from build123d import *

# Parameters (mm, degrees)
CHAMFER1_SIZE      = 0.508
CHAMFER2_SIZE      = 1.524
CUT_EXTRUDE1_DEPTH = 30.6672
FILLET1_R          = 0.762


with BuildPart() as part:
    # Sketch1 → Revolve1 (revolve)
    with BuildSketch(Plane.XY):
        with BuildLine():
            Line((0, 26.543), (0, -20.066))
            Line((0, -20.066), (-6.35, -20.066))
            Line((-6.35, -20.066), (-6.35, -3.81))
            Line((-6.35, -3.81), (-5.1943, -3.81))
            Line((-5.1943, -3.81), (-5.1943, -1.27))
            ThreePointArc((-5.1943, -1.27), (-5.566274388, -0.371974388), (-6.4643, 0))
            Line((-6.4643, 0), (-11.43, 0))
            Line((-11.43, 0), (-11.43, 9.6012))
            Line((-11.43, 9.6012), (-7.874, 9.6012))
            Line((-7.874, 9.6012), (-7.874, 17.0942))
            ThreePointArc((-7.874, 17.0942), (-6.35, 19.4056), (-7.874, 21.717))
            Line((-7.874, 21.717), (-7.874, 23.749))
            Line((-7.874, 23.749), (-5.08, 26.543))
            Line((-5.08, 26.543), (0, 26.543))
        make_face()
    revolve(axis=Axis((0, -20.066, 0), (0, -1, 0)))

    # Chamfer1
    chamfer1_edges = [part.edges().sort_by_distance(p)[0] for p in [
        (11.43, 9.6012, 0),
        (11.43, 0, 0),
    ]]
    chamfer(chamfer1_edges, length=CHAMFER1_SIZE)

    # Chamfer2
    chamfer2_edges = [part.edges().sort_by_distance(p)[0] for p in [
        (6.35, -20.066, 0),
    ]]
    chamfer(chamfer2_edges, length=CHAMFER2_SIZE)

    # Sketch2 → Cut-Extrude1 (cut, through all)
    with BuildSketch(Plane(origin=(0, 9.6012, 0), x_dir=(1, 0, 0), z_dir=(0, 1, 0))):
        with BuildLine():
            Line((-9.398, 6.505574225), (-9.398, -6.505574225))
            ThreePointArc((-9.398, -6.505574225), (-11.43, 0), (-9.398, 6.505574225))
        make_face()
        with BuildLine():
            Line((9.398, 6.505574225), (9.398, -6.505574225))
            ThreePointArc((9.398, -6.505574225), (11.43, 0), (9.398, 6.505574225))
        make_face()
    extrude(amount=-CUT_EXTRUDE1_DEPTH, mode=Mode.SUBTRACT)

    # Fillet1
    fillet1_edges = [part.edges().sort_by_distance(p)[0] for p in [
        (7.874, 9.6012, 0),
    ]]
    fillet(fillet1_edges, radius=FILLET1_R)


solid = part.part
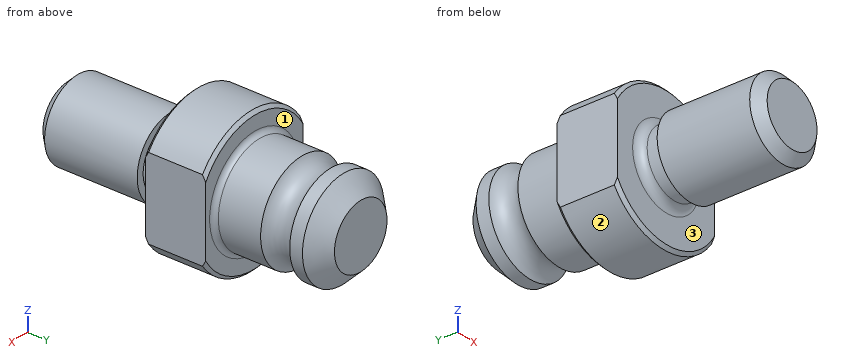
Design review of the part built by this model. Coordinates are the model's own, in mm. Face numbers are marked on the shaded views. A direction names the side the tool comes from. Coordinates: 2 decimals unless noted, no trailing zeros. Order: outer loops, then holes, each group sorted by start corner. A loop starts at its lowest first (then second) coordinate and runs counter-clockwise, first axis right, second up. Notation, with made-up numbers: M -33.75,40 L 15.25,40 A29 ccw 15.25,62 Z; hole C 85,30 d8. An arc over 180 degrees is marked long. Use a Markdown table: item, result.
(1) Add section C-C (y = -15.5). Give the boundary of the cut face in (x, z), then the cut area to 3 significant figures.
Worked answers:
| item | result |
|---|---|
| outline | C 0,0 d12.7 |
| area | 127 mm2 |
(2) Wall thickness on probe 1 along Y at (x, z) = (8, -5.5); probe 2 along Y at (x, z) = (-6.25, 0.75); probe 3 along Y at (x, z) = (3.5, 4): over which ranges is each line inside the solid? List them lowest first.
Worked answers:
| item | result |
|---|---|
| probe 1 | y = 0 to 9.6 |
| probe 2 | y = -18.6 to -3.81, -0.01 to 25.33 |
| probe 3 | y = -19.58 to -3.81, -0.73 to 26.31 |
(3) For P1, Ø8, axis at x = -4, y = -1.5, coming from the +Z side; P2, Ø1.5, axis at x = -7, z = -8, coming from the +Y side; P3, Ø1, axis at x = -4.5, z = -7, coming from the -Y side, all flat-tipped, find the tip position at first contact; note any pin that passes through.
Worked answers:
| item | result |
|---|---|
| P1 | stops at z = 11.42 |
| P2 | stops at y = 9.6 |
| P3 | stops at y = 0 |
(4) For the marked faces 1, 2 and 3, list the 3-axis set-ups (+Z, -Z, +X, -X, +Y, -Y) from which the entire face can be reached by the end or side of a thin tool; tool diameter is ignored.
Worked answers:
| item | result |
|---|---|
| face 1 | +Y |
| face 2 | -Z, +Y, -Y |
| face 3 | -Y |
(5) Add section B-B (z = 0). Give the boundary of the cut face in (x, y).
Worked answers:
| item | result |
|---|---|
| outline | M -9.4,0 L -6.46,0 A1.27 cw -5.19,-1.27 L -5.19,-3.81 L -6.35,-3.81 L -6.35,-18.54 L -4.83,-20.07 L 4.83,-20.07 L 6.35,-18.54 L 6.35,-3.81 L 5.19,-3.81 L 5.19,-1.27 A1.27 cw 6.46,0 L 9.4,0 L 9.4,9.6 L 8.64,9.6 A0.76 cw 7.87,10.36 L 7.87,17.09 A2.51 cw 7.87,21.72 L 7.87,23.75 L 5.08,26.54 L -5.08,26.54 L -7.87,23.75 L -7.87,21.72 A2.51 cw -7.87,17.09 L -7.87,10.36 A0.76 cw -8.64,9.6 L -9.4,9.6 Z |
(6) Add section D-D (y = 6). Give the boundary of the cut face in (x, z).
Worked answers:
| item | result |
|---|---|
| outline | M -9.4,-6.51 A11.43 ccw 9.4,-6.51 L 9.4,6.51 A11.43 ccw -9.4,6.51 Z |
